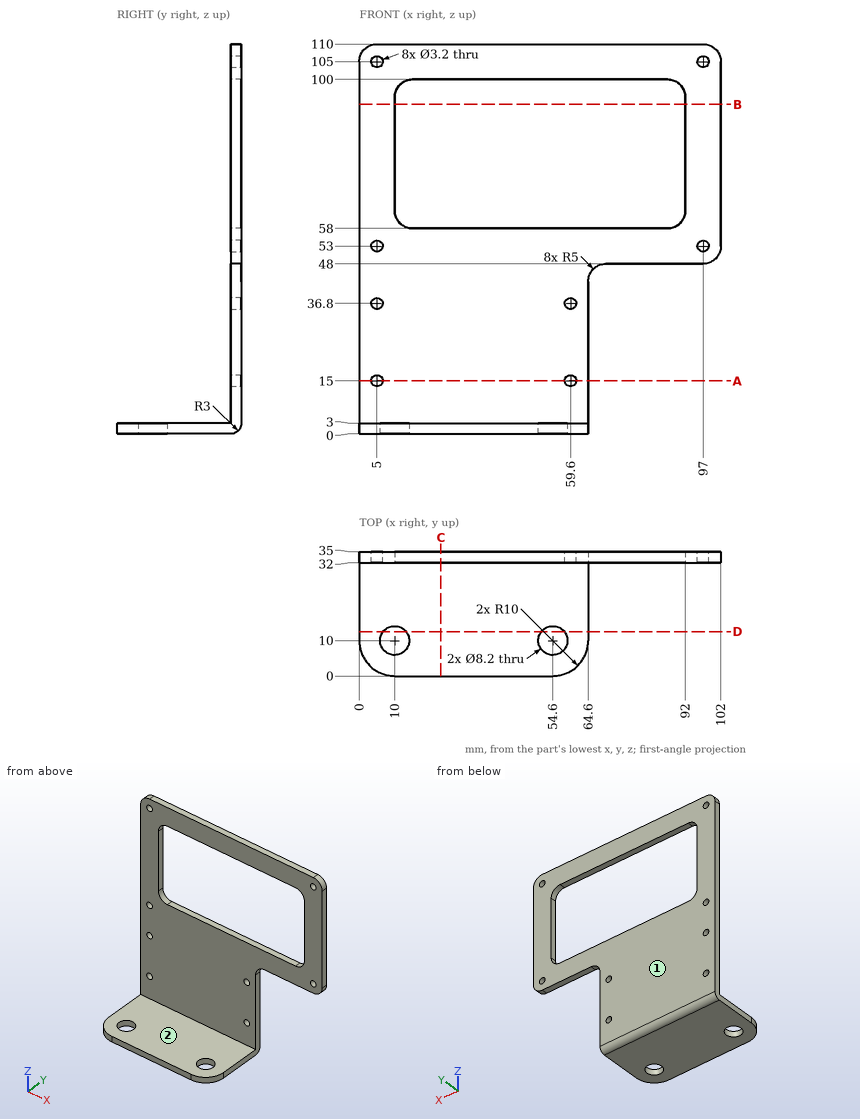
Could you check a few things on this drawing? It's one solid part, dimensions in mm from its lowest x, y, z. A direction names the side the tool comes from. Round coordinates to 2 decimals unless told otherwise and drop trailing zeros. Order: outer loops, then holes, each group sorted by start corner. A loop starts at its lowest first (then second) coordinate and runs counter-clockwise, first axis right, second up. Notation, with made-up numbers: M -7.75,81.5 L 42.25,81.5 A27 cw 42.25,100.5 Z; hole C 60.5,-20.5 d7. An arc over 180 degrees is marked long. One line per question, with ' | ' between items. Start each with the question number.
(1) Suppose I cut it at B-B on z = 93. List the corners of the cut face in (x, y) for me.
(2) Suppose I cut it at D-D on y = 12.5. List the corners of the cut face in (x, z) for me.
(3) Please list where these lines run through material, in increasing order: line 1 along X through (y, z) = (33, 15); line 2 along X through (y, z) = (34.45, 105); line 3 along Y through (x, z) = (55, 38.5).
(4) Suppose I cut it at A-A on z = 15. List the corners of the cut face in (x, y) for me, then the cut area to 3 significant figures.
(5) For P1, Ø0.9, axis at x = 47.5, y = 34, coming from the -Z side; P2, Ø4, axis at x = 5, z = 53, coming from the +Y side; P3, Ø6, axis at x = 15.5, y = 20.5, coming from the +Z side; P4, Ø3.5, axis at x = 84, y = 34, coming from the -Z side, each with a flat end and sliding along its axis, tell me the tip position at first contact or that it passes through.
(6) Suppose I cut it at C-C on x = 23. List the corners of the cut face in (y, z) for me.
(7) For the marked faces 1 and 2, which set-ups out of +Z, -Z, +X, -X, +Y, -Y let a thin tool reach every point of the face, with its end or its side?
Geometry results:
1) outline: M 0,32 L 10,32 L 10,35 L 0,35 Z; M 92,32 L 102,32 L 102,35 L 92,35 Z
2) outline: M 0,0 L 6.75,0 L 6.75,3 L 0,3 Z; M 13.25,0 L 51.35,0 L 51.35,3 L 13.25,3 Z; M 57.85,0 L 64.6,0 L 64.6,3 L 57.85,3 Z
3) line 1: 0 to 3.4, 6.6 to 58, 61.2 to 64.6 | line 2: 0 to 3.4, 6.6 to 95.4, 98.6 to 102 | line 3: 32 to 35
4) outline: M 0,32 L 3.4,32 L 3.4,35 L 0,35 Z; M 6.6,32 L 58,32 L 58,35 L 6.6,35 Z; M 61.2,32 L 64.6,32 L 64.6,35 L 61.2,35 Z | area: 175 mm²
5) P1: z = 0.43 | P2: y = 35 | P3: z = 3 | P4: z = 48
6) outline: M 0,0 L 32,0 A3 ccw 35,3 L 35,58 L 32,58 L 32,3 L 0,3 Z; M 32,100 L 35,100 L 35,110 L 32,110 Z
7) face 1: +Z, -Z, +X, -X, +Y | face 2: +Z, +X, -X, -Y
